Part print with two shaded views. Sizes in mm from the minimum x, y, z corner. Coordinates: 2 decimals unless noted, no trailing zeros. Loops run counter-clockwise (first coordinate to the right, second up) from the corner with the lowest first, then second, coordinate; pieces in that order, holes last. Notation, with made-up numbers: (34, 60) -> (40, 60) arc R4 cw to (40, 66) -> close; hole circle Ø1 at (84, 66.25). An arc over 180 degrees is marked (long way). Write each question's results on one line, items separated by ' | '.
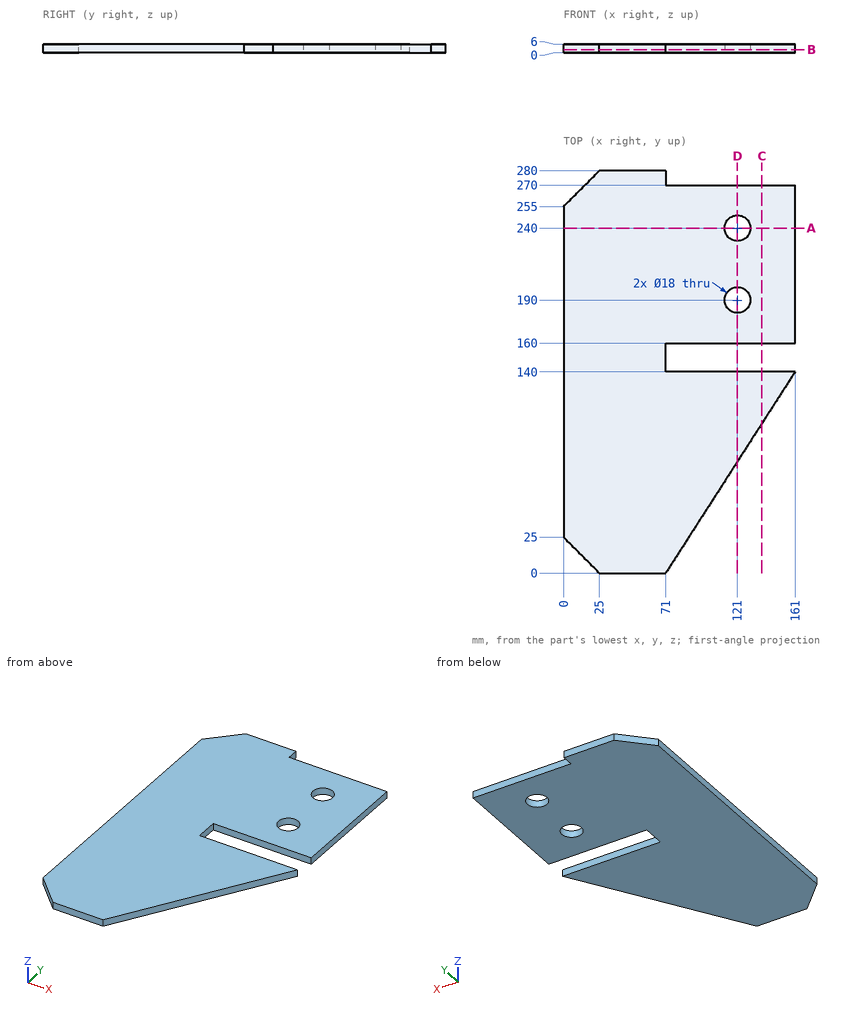
Q1. Cut at A-A on y = 240. Write the cut outline in (x, z), and give its area (3 significant figures).
Results are:
outline: (0, 0) -> (112, 0) -> (112, 6) -> (0, 6) -> close; (130, 0) -> (161, 0) -> (161, 6) -> (130, 6) -> close | area: 858 mm^2
Q2. Drop flat-ended pins along their axis: pin 1 (14.5 mm diameter, centred on x = 121, y = 240, fed in from -Z); pin 2 (3 mm diameter, centred on x = 137, z = 1.5, fed in from +Y); pin 3 (1.8 mm diameter, centred on y = 154.5, z = 3.5, fed in from +X). Give the stop position or say it passes through.
Results are:
pin 1: through | pin 2: y = 270 | pin 3: x = 71
Q3. Cut at C-C on x = 138. Write the cut outline in (y, z), and give its area (3 significant figures).
Results are:
outline: (104.22, 0) -> (140, 0) -> (140, 6) -> (104.22, 6) -> close; (160, 0) -> (270, 0) -> (270, 6) -> (160, 6) -> close | area: 875 mm^2
Q4. Wall check: L1, parallel to X at y = 190, z = 4.15; L2, parallel to Y at x = 121, z = 2.05; L3, parallel to Y at x = 105, z = 3.6. Give the ranges that are in metal, low to high. Write a range as from..to.
Results are:
L1: 0..112, 130..161 | L2: 77.78..140, 160..181, 199..231, 249..270 | L3: 52.89..140, 160..270
Q5. Cut at D-D on x = 121. Write the cut outline in (y, z), and give its area (3 significant figures).
Results are:
outline: (77.78, 0) -> (140, 0) -> (140, 6) -> (77.78, 6) -> close; (160, 0) -> (181, 0) -> (181, 6) -> (160, 6) -> close; (199, 0) -> (231, 0) -> (231, 6) -> (199, 6) -> close; (249, 0) -> (270, 0) -> (270, 6) -> (249, 6) -> close | area: 817 mm^2
Q6. Cut at B-B on z = 2.05. Write the cut outline in (x, y).
Results are:
outline: (0, 25) -> (25, 0) -> (71, 0) -> (161, 140) -> (71, 140) -> (71, 160) -> (161, 160) -> (161, 270) -> (71, 270) -> (71, 280) -> (25, 280) -> (0, 255) -> close; hole circle Ø18 at (121, 190); hole circle Ø18 at (121, 240)
